from build123d import *

# Parameters (mm, degrees)
F0_R         = 30
F1_DEPTH     = 2
F2_R         = 27.95
F3_DEPTH     = 7
F4_T         = -2
F5_W         = 13
F5_H         = 10
F6_DEPTH     = 30
F7_T1_DEPTH  = 7.3004746493
F7_T3_DEPTH  = 6.5918643954
F7_T5_DEPTH  = 6.4134609486
F7_T7_DEPTH  = 7.0163816712
F7_T12_ANGLE = 11.2783830284
F7_T17_ANGLE = 20.9875744089
F7_T22_ANGLE = 22.6619870068
F7_T27_ANGLE = 12.1533364168
F7_T30_ANGLE = 338.3067764097
F7_T35_ANGLE = 11.2783830284
F7_T39_DEPTH = 7.0163816712
F7_T47_DEPTH = 7.3004746493
F7_T52_ANGLE = 20.9875744089
F7_T59_ANGLE = 22.6619870068
F7_T63_DEPTH = 6.4134609486
F7_T70_ANGLE = 12.1533364168
F7_T74_DEPTH = 6.5918643954
F8_R         = 4.5
F9_DEPTH     = 25


# Not quite as in the source:
# - a fillet or chamfer that OpenCascade refuses, or shapes differently, is made with other operations: its cross-section is extruded or revolved along the edge and cut away or added


with BuildPart() as f1:
    # F0 (on Top) → F1 (new body)
    with BuildSketch(Plane.XY):
        Circle(F0_R)
    extrude(amount=F1_DEPTH)

    # F2 (on face) → F3 (join)
    with BuildSketch(Plane(origin=(0, 0, 0), x_dir=(1, 0, 0), z_dir=(0, 0, -1))):
        Circle(F2_R)
    extrude(amount=F3_DEPTH)

    # F4
    f4_openings = [f1.faces().sort_by_distance(p)[0] for p in [
        (0, 0, -7),
    ]]
    offset(amount=F4_T, openings=f4_openings, kind=Kind.INTERSECTION)

    # F5 (on Right) → F6 (cut)
    with BuildSketch(Plane.YZ):
        with Locations((-2.3, -6.5)):
            Rectangle(F5_W, F5_H)
    extrude(amount=F6_DEPTH, mode=Mode.SUBTRACT)

    # F7: chamfer of 0.5 on 9 edges, made by hand

    # F7_s2 → F7_t1 (cut)
    with BuildSketch(Plane.XY.offset(-8.8004746493)):
        with BuildLine():
            Line((26.2970147419, -9.4693989071), (25.8265851401, -8.8))
            Line((25.8265851401, -8.8), (26.5285223863, -8.8))
            ThreePointArc((26.5285223863, -8.8), (26.4129758895, -9.1409630052), (26.2970147419, -9.4693989071))
        make_face()
    extrude(amount=F7_T1_DEPTH, mode=Mode.SUBTRACT)

    # F7_s4 → F7_t3 (cut)
    with BuildSketch(Plane.XY.offset(-8.0918643954)):
        with BuildLine():
            Line((26.0290702869, 4.2), (25.5370273703, 4.6111531191))
            ThreePointArc((25.5370273703, 4.6111531191), (25.5719745626, 4.4132320321), (25.6078601215, 4.2))
            Line((25.6078601215, 4.2), (26.0290702869, 4.2))
        make_face()
    extrude(amount=F7_T3_DEPTH, mode=Mode.SUBTRACT)

    # F7_s6 → F7_t5 (cut)
    with BuildSketch(Plane.XY.offset(-7.9134609486)):
        with BuildLine():
            Line((24.7611086182, -8.8), (24.2930347312, -9.1241965974))
            ThreePointArc((24.2930347312, -9.1241965974), (24.3504005172, -8.9699774052), (24.4123431895, -8.8))
            Line((24.4123431895, -8.8), (24.7611086182, -8.8))
        make_face()
    extrude(amount=F7_T5_DEPTH, mode=Mode.SUBTRACT)

    # F7_s8 → F7_t7 (cut)
    with BuildSketch(Plane.XY.offset(-8.5163816712)):
        with BuildLine():
            Line((27.5372554008, 4.7856102004), (27.0446390251, 4.2))
            Line((27.0446390251, 4.2), (27.6326346916, 4.2))
            ThreePointArc((27.6326346916, 4.2), (27.585450674, 4.4994900946), (27.5372554008, 4.7856102004))
        make_face()
    extrude(amount=F7_T7_DEPTH, mode=Mode.SUBTRACT)


with BuildPart() as f7_tool10:
    # F7_s11 → F7_t12 (revolve)
    with BuildSketch(Plane.XZ):
        Polygon((27.95, -1), (27.45, -1.5), (27.95, -1.5), align=None)
    revolve(axis=Axis((0, 0, -1.5), (0, 0, 1)), revolution_arc=F7_T12_ANGLE)

    split(bisect_by=Plane.XZ.offset(-4.2), keep=Keep.TOP)


with BuildPart() as f1_1:
    add(f1.part)

    # F7_t9: cut F7_tool10
    add(f7_tool10.part, mode=Mode.SUBTRACT)


with BuildPart() as f7_tool15:
    # F7_s16 → F7_t17 (revolve)
    with BuildSketch(Plane(origin=(0, 0, 0), x_dir=(0, 0, 1), z_dir=(-0.3581654779, -0.9336581229, 0))):
        Polygon((-1, -27.95), (-1.5, -27.45), (-1.5, -27.95), align=None)
    revolve(axis=Axis((0, 0, -1.5), (0, 0, 1)), revolution_arc=F7_T17_ANGLE)

    split(bisect_by=Plane.XZ.offset(8.8), keep=Keep.BOTTOM)


with BuildPart() as f1_2:
    add(f1_1.part)

    # F7_t14: cut F7_tool15
    add(f7_tool15.part, mode=Mode.SUBTRACT)


with BuildPart() as f7_tool20:
    # F7_s21 → F7_t22 (revolve)
    with BuildSketch(Plane(origin=(0, 0, 0), x_dir=(0, 0, 1), z_dir=(-0.3852938978, -0.9227939165, 0))):
        Polygon((-1.5, -26.45), (-1, -25.95), (-1.5, -25.95), align=None)
    revolve(axis=Axis((0, 0, -1.5), (0, 0, 1)), revolution_arc=F7_T22_ANGLE)

    split(bisect_by=Plane.XZ.offset(8.8), keep=Keep.BOTTOM)


with BuildPart() as f1_3:
    add(f1_2.part)

    # F7_t19: cut F7_tool20
    add(f7_tool20.part, mode=Mode.SUBTRACT)


with BuildPart() as f7_tool25:
    # F7_s26 → F7_t27 (revolve)
    with BuildSketch(Plane.XZ):
        Polygon((26.45, -1.5), (25.95, -1), (25.95, -1.5), align=None)
    revolve(axis=Axis((0, 0, -1.5), (0, 0, 1)), revolution_arc=F7_T27_ANGLE)

    split(bisect_by=Plane.XZ.offset(-4.2), keep=Keep.TOP)


with BuildPart() as f1_4:
    add(f1_3.part)

    # F7_t24: cut F7_tool25
    add(f7_tool25.part, mode=Mode.SUBTRACT)

    # F7_s29 → F7_t30 (revolve, cut)
    with BuildSketch(Plane(origin=(0, 0, 0), x_dir=(0, 0, 1), z_dir=(0.2706204465, 0.9626861243, 0))):
        Polygon((-6.5, 27.95), (-7, 27.45), (-7, 27.95), align=None)
    revolve(axis=Axis((0, 0, -7), (0, 0, -1)), revolution_arc=F7_T30_ANGLE, mode=Mode.SUBTRACT)


with BuildPart() as f7_tool33:
    # F7_s34 → F7_t35 (revolve)
    with BuildSketch(Plane.XZ):
        Polygon((27.95, -1), (27.45, -1.5), (27.95, -1.5), align=None)
    revolve(axis=Axis((0, 0, -1.5), (0, 0, 1)), revolution_arc=F7_T35_ANGLE)

    split(bisect_by=Plane.XZ.offset(-4.2), keep=Keep.BOTTOM)


with BuildPart() as f7_tool37:
    # F7_s38 → F7_t39 (new body)
    with BuildSketch(Plane.XY.offset(-7)):
        with BuildLine():
            Line((27.5372554008, 4.7856102004), (27.0446390251, 4.2))
            Line((27.0446390251, 4.2), (27.6326346916, 4.2))
            ThreePointArc((27.6326346916, 4.2), (27.585450674, 4.4994900946), (27.5372554008, 4.7856102004))
        make_face()
    extrude(amount=F7_T39_DEPTH)

    split(bisect_by=Plane.XY, keep=Keep.BOTTOM)

    split(bisect_by=Plane.XY.offset(-1.5), keep=Keep.TOP)


with BuildPart() as f7_tool33_1:
    add(f7_tool33.part)

    # F7_t42: intersect F7_tool37
    add(f7_tool37.part, mode=Mode.INTERSECT)


with BuildPart() as f1_5:
    add(f1_4.part)

    # F7_t31: cut F7_tool33
    add(f7_tool33_1.part, mode=Mode.SUBTRACT)


with BuildPart() as f7_tool45:
    # F7_s46 → F7_t47 (new body)
    with BuildSketch(Plane.XY.offset(-7)):
        with BuildLine():
            Line((26.2970147419, -9.4693989071), (25.8265851401, -8.8))
            Line((25.8265851401, -8.8), (26.5285223863, -8.8))
            ThreePointArc((26.5285223863, -8.8), (26.4129758895, -9.1409630052), (26.2970147419, -9.4693989071))
        make_face()
    extrude(amount=F7_T47_DEPTH)

    split(bisect_by=Plane.XY, keep=Keep.BOTTOM)

    split(bisect_by=Plane.XY.offset(-1.5), keep=Keep.TOP)


with BuildPart() as f7_tool50:
    # F7_s51 → F7_t52 (revolve)
    with BuildSketch(Plane(origin=(0, 0, 0), x_dir=(0, 0, 1), z_dir=(-0.3581654779, -0.9336581229, 0))):
        Polygon((-1, -27.95), (-1.5, -27.45), (-1.5, -27.95), align=None)
    revolve(axis=Axis((0, 0, -1.5), (0, 0, 1)), revolution_arc=F7_T52_ANGLE)

    split(bisect_by=Plane.XZ.offset(8.8), keep=Keep.TOP)


with BuildPart() as f7_tool45_1:
    add(f7_tool45.part)

    # F7_t54: intersect F7_tool50
    add(f7_tool50.part, mode=Mode.INTERSECT)


with BuildPart() as f1_6:
    add(f1_5.part)

    # F7_t43: cut F7_tool45
    add(f7_tool45_1.part, mode=Mode.SUBTRACT)


with BuildPart() as f7_tool57:
    # F7_s58 → F7_t59 (revolve)
    with BuildSketch(Plane(origin=(0, 0, 0), x_dir=(0, 0, 1), z_dir=(-0.3852938978, -0.9227939165, 0))):
        Polygon((-1.5, -26.45), (-1, -25.95), (-1.5, -25.95), align=None)
    revolve(axis=Axis((0, 0, -1.5), (0, 0, 1)), revolution_arc=F7_T59_ANGLE)

    split(bisect_by=Plane.XZ.offset(8.8), keep=Keep.TOP)


with BuildPart() as f7_tool61:
    # F7_s62 → F7_t63 (new body)
    with BuildSketch(Plane.XY.offset(-7)):
        with BuildLine():
            Line((24.7611086182, -8.8), (24.2930347312, -9.1241965974))
            ThreePointArc((24.2930347312, -9.1241965974), (24.3504005172, -8.9699774052), (24.4123431895, -8.8))
            Line((24.4123431895, -8.8), (24.7611086182, -8.8))
        make_face()
    extrude(amount=F7_T63_DEPTH)

    split(bisect_by=Plane.XY.offset(-1.5), keep=Keep.TOP)


with BuildPart() as f7_tool57_1:
    add(f7_tool57.part)

    # F7_t65: intersect F7_tool61
    add(f7_tool61.part, mode=Mode.INTERSECT)


with BuildPart() as f1_7:
    add(f1_6.part)

    # F7_t55: cut F7_tool57
    add(f7_tool57_1.part, mode=Mode.SUBTRACT)


with BuildPart() as f7_tool68:
    # F7_s69 → F7_t70 (revolve)
    with BuildSketch(Plane.XZ):
        Polygon((26.45, -1.5), (25.95, -1), (25.95, -1.5), align=None)
    revolve(axis=Axis((0, 0, -1.5), (0, 0, 1)), revolution_arc=F7_T70_ANGLE)

    split(bisect_by=Plane.XZ.offset(-4.2), keep=Keep.BOTTOM)


with BuildPart() as f7_tool72:
    # F7_s73 → F7_t74 (new body)
    with BuildSketch(Plane.XY.offset(-7)):
        with BuildLine():
            Line((26.0290702869, 4.2), (25.5370273703, 4.6111531191))
            ThreePointArc((25.5370273703, 4.6111531191), (25.5719745626, 4.4132320321), (25.6078601215, 4.2))
            Line((25.6078601215, 4.2), (26.0290702869, 4.2))
        make_face()
    extrude(amount=F7_T74_DEPTH)

    split(bisect_by=Plane.XY.offset(-1.5), keep=Keep.TOP)


with BuildPart() as f7_tool68_1:
    add(f7_tool68.part)

    # F7_t76: intersect F7_tool72
    add(f7_tool72.part, mode=Mode.INTERSECT)


with BuildPart() as f1_8:
    add(f1_7.part)

    # F7_t66: cut F7_tool68
    add(f7_tool68_1.part, mode=Mode.SUBTRACT)

    # F8 (on face) → F9 (cut)
    with BuildSketch(Plane.XY):
        with Locations((19.798791036, -14.3004134297)):
            Circle(F8_R)
        with Locations((-19.798791036, -14.3004134297)):
            Circle(F8_R)
        with Locations((19.798791036, 14.3004134297)):
            Circle(F8_R)
        with Locations((-19.798791036, 14.3004134297)):
            Circle(F8_R)
    extrude(amount=-F9_DEPTH, mode=Mode.SUBTRACT)


solid = f1_8.part
Part model, mm, in its own coordinate system. A direction names the side the tool comes from. Round coordinates to 2 decimals unless told otherwise and drop trailing zeros. Write each loop counter-clockwise with the first axis right and the second up, starting at its lowest first coordinate (ties: lowest second). Pieces come first, ordered by that corner, then holes. Notation, with made-up numbers: (88, 12.5) - (96, 12.5) arc R36 ccw to (96, 50.5) - close; hole circle Ø4 at (58, -35.5). An arc over 180 degrees is marked (long way). Use CSV: the item, a comma, the result in double quotes.
Item 1: Slice it at A-A, the plane z = -3.75. Write the cut outline in (x, y), then the cut area to 3 significant figures.
Results list:
outline,"(-24.28, -13.85) arc R4.5 cw to (-23.28, -11.45) arc R25.95 cw to (-23.28, 11.45) arc R4.5 cw to (-24.28, 13.85) arc R27.95 ccw to start; (-20.78, -18.69) arc R27.95 ccw to (20.78, -18.69) arc R4.5 cw to (18.19, -18.5) arc R25.95 cw to (-18.19, -18.5) arc R4.5 cw to start; (-20.78, 18.69) arc R4.5 cw to (-18.19, 18.5) arc R25.95 cw to (18.19, 18.5) arc R4.5 cw to (20.78, 18.69) arc R27.95 ccw to start; (23.28, -11.45) arc R4.5 cw to (24.28, -13.85) arc R27.95 ccw to (26.3, -9.47) - (25.83, -8.8) - (24.76, -8.8) - (24.29, -9.12) arc R25.95 cw to start; (23.28, 11.45) arc R25.95 cw to (25.54, 4.61) - (26.03, 4.2) - (27.04, 4.2) - (27.54, 4.79) arc R27.95 ccw to (24.28, 13.85) arc R4.5 cw to start"
area,"250 mm²"
Item 2: Flat gauge pins, fed straight in: P1, Ø0.8, axis at x = 26, y = -4.5, coming from the -Z side; P2, Ø4, axis at x = -13, y = -3, coming from the -Z side; P3, Ø5, axis at y = -1.5, z = -4, coming from the -X side. Where does each tip first touch, or does it go through?
Results list:
P1,"stops at z = -1.5"
P2,"stops at z = 0"
P3,"stops at x = -27.95"
Item 3: Pull direction X, two halves, no side cores. Call faces 6 (the flat face through (-26.3, -0.2, -7)), 7 (the cylindrical face through (-27.95, -0.2, -3.2)), 8 (the cylindrical face through (-19.454, 18.787, -3.451)), 9 (the conical face through (26.058, 9.221, -6.809)): pulls with the +X half, pulls with the -X half, needs draft (parallel to the pull), parting line crosses it, or undercut.
Results list:
face 6,"needs draft"
face 7,"pulls with the -X half"
face 8,"undercut"
face 9,"pulls with the +X half"
Item 4: Tool access for faces 1 (the cylindrical face through (27.74, 3.41, -0.32)), 2 (the cylindrical face through (0.33, -27.95, -3.2)), 3 (the conical face through (25.97, -2.451, -1.135)), 4 (the cylindrical face through (23.95, 12.56, -3.45)), 5 (the conical face through (25.24, -11.403, -6.753)): list every direction of +Z, -Z, +X, -X, +Y, -Y with a clear straight run to the whole face (end or side of a thin tool).
Results list:
face 1,"-Z, +X"
face 2,"-Z, -Y"
face 3,"-Z"
face 4,"-Z, +Y"
face 5,"-Z, +X, -Y"
Item 5: Wall check: L1, parallel to Y at x = -19.5, z = -1.75; L2, parallel to X at y = 0.5, z = -4.5; L3, parallel to Z at x = 20, y = -5. Give the ranges that are in metal, low to high.
Results list:
L1,"y = -20.02 to -18.79, 18.79 to 20.02"
L2,"x = -27.95 to -25.95"
L3,"z = 0 to 2"
Item 6: Slice it at D-D, the plane y = 17.5. Write the cut outline in (x, z).
Results list:
outline,"(-24.37, 0) - (24.37, 0) - (24.37, 2) - (-24.37, 2) - close"
Item 7: Slice it at B-B, the plane x = 0. Write the cut outline in (y, z), then the cut area to 3 significant figures.
Results list:
outline,"(-30, 0) - (-27.95, 0) - (-27.95, -6.5) - (-27.45, -7) - (-25.95, -7) - (-25.95, 0) - (25.95, 0) - (25.95, -7) - (27.45, -7) - (27.95, -6.5) - (27.95, 0) - (30, 0) - (30, 2) - (-30, 2) - close"
area,"148 mm²"
Item 8: Slice it at C-C, the plane y = 0. Write the cut outline in (x, z), then the cut area to 3 significant figures.
Results list:
outline,"(-30, 0) - (-27.95, 0) - (-27.95, -6.5) - (-27.45, -7) - (-25.95, -7) - (-25.95, 0) - (25.95, 0) - (25.95, -1) - (26.45, -1.5) - (27.45, -1.5) - (27.95, -1) - (27.95, 0) - (30, 0) - (30, 2) - (-30, 2) - close"
area,"137 mm²"
